```python
from build123d import *

# Parameters (mm, degrees)
SKETCH1_R           = 2.1
SKETCH1_R_2         = 1.5
SKETCH1_W           = 42
SKETCH1_H           = 21
BOSS_EXTRUDE1_DEPTH = 10
BOSS_EXTRUDE2_START = -30
BOSS_EXTRUDE2_DEPTH = 30
SKETCH3_W           = 75
SKETCH3_H           = 8
CUT_EXTRUDE1_DEPTH  = 45
SKETCH4_W           = 7.58
SKETCH4_H           = 21
CUT_EXTRUDE2_DEPTH  = 3


with BuildPart() as part:
    # Sketch1 → Boss-Extrude1 (new body)
    with BuildSketch(Plane(origin=(0, 0, 0), x_dir=(1, 0, 0), z_dir=(0, 1, 0))):
        with BuildLine():
            Line((-100, 32.5), (100, 32.5))
            ThreePointArc((100, 32.5), (132.5, 0), (100, -32.5))
            Line((100, -32.5), (-100, -32.5))
            ThreePointArc((-100, -32.5), (-132.5, 0), (-100, 32.5))
        make_face()
        with Locations(Location((-115.5, 4.9, 0), (0, 0, 270))):
            Circle(SKETCH1_R, mode=Mode.SUBTRACT)
        with Locations(Location((-115.5, -4.9, 0), (0, 0, 270))):
            Circle(SKETCH1_R, mode=Mode.SUBTRACT)
        with Locations(Location((-66.5, -4.9, 0), (0, 0, 270))):
            Circle(SKETCH1_R, mode=Mode.SUBTRACT)
        with Locations(Location((-66.5, 4.9, 0), (0, 0, 270))):
            Circle(SKETCH1_R, mode=Mode.SUBTRACT)
        with Locations(Location((85, 15, 0), (0, 0, 270))):
            Circle(SKETCH1_R_2, mode=Mode.SUBTRACT)
        with Locations(Location((115, 15, 0), (0, 0, 90))):
            Circle(SKETCH1_R_2, mode=Mode.SUBTRACT)
        with Locations(Location((85, -15, 0), (0, 0, 90))):
            Circle(SKETCH1_R_2, mode=Mode.SUBTRACT)
        with Locations(Location((115, -15, 0), (0, 0, 270))):
            Circle(SKETCH1_R_2, mode=Mode.SUBTRACT)
        with Locations((-91, 0)):
            Rectangle(SKETCH1_W, SKETCH1_H, mode=Mode.SUBTRACT)
        Polygon((0, 21.5), (-40, 21.5), (-40, 12), (0, 12), (50, 12), (50, 21.5), align=None, mode=Mode.SUBTRACT)
        Polygon((-50, 4.75), (0, 4.75), (65, 4.75), (65, -4.75), (0, -4.75), (-50, -4.75), align=None, mode=Mode.SUBTRACT)
        Polygon((0, -12), (-40, -12), (-40, -21.5), (0, -21.5), (50, -21.5), (50, -12), align=None, mode=Mode.SUBTRACT)
    extrude(amount=BOSS_EXTRUDE1_DEPTH)

    # Sketch2 → Boss-Extrude2 (add)
    with BuildSketch(Plane(origin=(0, 0, 0), x_dir=(1, 0, 0), z_dir=(0, 1, 0)).offset(BOSS_EXTRUDE2_START)):
        with BuildLine():
            Line((-100, 32.5), (100, 32.5))
            ThreePointArc((100, 32.5), (132.5, 0), (100, -32.5))
            Line((100, -32.5), (-100, -32.5))
            ThreePointArc((-100, -32.5), (-132.5, 0), (-100, 32.5))
        make_face()
        with BuildLine():
            Line((99.668543355, 27.510998447), (-100, 27.510998447))
            ThreePointArc((-100, 27.510998447), (-127.55585262, -0.044854173), (-100, -27.600706793))
            Line((-100, -27.600706793), (100.998461852, -27.600706793))
            ThreePointArc((100.998461852, -27.600706793), (128.562336478, 0.636345006), (99.668543355, 27.510998447))
        make_face(mode=Mode.SUBTRACT)
    extrude(amount=BOSS_EXTRUDE2_DEPTH)

    # Sketch3 → Cut-Extrude1 (cut, symmetric)
    with BuildSketch(Plane.XY):
        with Locations((-57.5, -19)):
            Rectangle(SKETCH3_W, SKETCH3_H)
        with Locations((57.5, -19)):
            Rectangle(SKETCH3_W, SKETCH3_H)
        with Locations((57.5, -4)):
            Rectangle(SKETCH3_W, SKETCH3_H)
        with Locations((-57.5, -4)):
            Rectangle(SKETCH3_W, SKETCH3_H)
    extrude(amount=CUT_EXTRUDE1_DEPTH, both=True, mode=Mode.SUBTRACT)

    # Sketch4 → Cut-Extrude2 (cut)
    with BuildSketch(Plane(origin=(0, 10, 0), x_dir=(1, 0, 0), z_dir=(0, 1, 0))):
        with Locations((-115.79, 0)):
            Rectangle(SKETCH4_W, SKETCH4_H)
        with Locations((-66.21, 0)):
            Rectangle(SKETCH4_W, SKETCH4_H)
    extrude(amount=-CUT_EXTRUDE2_DEPTH, mode=Mode.SUBTRACT)


solid = part.part
```
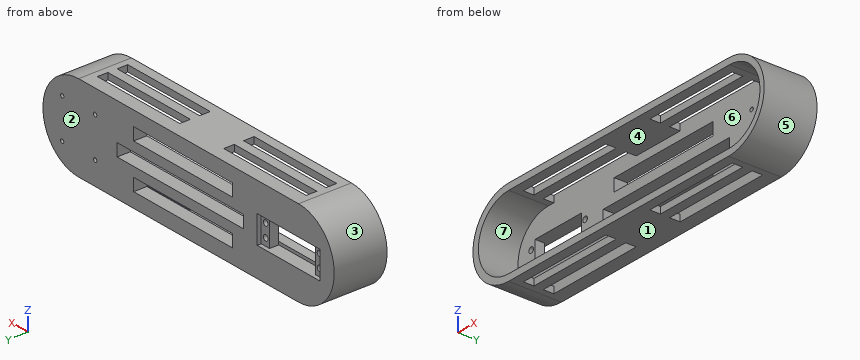
The model under review builds one solid part; all positions refer to its coordinate system, in mm. Face numbers are marked on the shaded views. A direction names the side the tool comes from. Round coordinates to 2 decimals unless told otherwise and drop trailing zeros. Loops run counter-clockwise (first coordinate to the right, second up) from the corner with the lowest first, then second, coordinate; pieces in that order, holes last. Notation, with made-up numbers: (-24, 85) - (32, 85) arc R30 ccw to (32, 109) - close; hole circle Ø6 at (9, 49.25). An arc over 180 degrees is marked (long way). Write each question's results on one line, items separated by ' | '. Start each with the question number.
Q1. Wall thickness on line 1 along Y through (x, z) = (-71, -28); line 2 along Z through (x, y) = (85, 7); line 3 along Z through (x, y) = (-58.5, -14): over which ranges is each line inside the solid? List them lowest first. Write a range as [from, to].
Q2. Draft analysis for pull direction Z (two halves, no side actions). For the marked faces 1, 2, 3 and 4, state which applies: pulls with the +Z half, pulls with the -Z half, needs draft (parallel to the pull), parting line crosses it, or undercut.
Q3. Take a section at C-C on z = 0. Give the boundary of the cut face in (x, y), plus the area to 3 significant figures.
Q4. Take a section at B-B on x = 4.5. Give the boundary of the cut face in (y, z), plus the area to 3 significant figures.
Q5. Insertion check: P1, Ø3, axis at y = 4.5, z = -17.5, coming from the +X side; P2, Ø10, axis at y = -22, z = 23.5, coming from the -X side; P3, Ø2.5, axis at y = -17, z = 29, coming from the +X side. Each pin has a flat end and moves straight along its axis. Give the tip position at first contact, or say it passes through.
Q6. Take a section at A-A on x = 56. Give the boundary of the cut face in (y, z), plus the area to 3 significant figures.
Q7. Tool access review of the marked faces 5, 6 and 7: name each direction out of +Z, -Z, +X, -X, +Y, -Y from which nothing blocks a thin tool from reaching the whole face with its end or side.
Data:
1) line 1: y = [-30, -23], [-15, -8], [0, 10] | line 2: z = [-32.5, -16.5], [-13.5, 13.5], [16.5, 32.5] | line 3: z = [-32.5, -27.51], [27.6, 32.5]
2) face 1: pulls with the -Z half | face 2: needs draft | face 3: parting line crosses it | face 4: undercut
3) outline: (-132.5, -30) - (-127.56, -30) - (-127.56, 0) - (-112, 0) - (-112, 7) - (-119.58, 7) - (-119.58, 10) - (-132.5, 10) - close; (-70, 0) - (-50, 0) - (-50, 10) - (-62.42, 10) - (-62.42, 7) - (-70, 7) - close; (65, 0) - (128.57, 0) - (128.57, -30) - (132.5, -30) - (132.5, 10) - (65, 10) - close | area: 1,300 mm²
4) outline: (-30, -32.5) - (10, -32.5) - (10, -21.5) - (0, -21.5) - (0, -27.51) - (-30, -27.51) - close; (-30, 27.6) - (0, 27.6) - (0, 21.5) - (10, 21.5) - (10, 32.5) - (-30, 32.5) - close; (0, -12) - (10, -12) - (10, -4.75) - (0, -4.75) - close; (0, 4.75) - (10, 4.75) - (10, 12) - (0, 12) - close | area: 662 mm²
5) P1: stops at x = 128.29 | P2: stops at x = -126.72 | P3: stops at x = 116.92
6) outline: (-30, -32.5) - (-23, -32.5) - (-23, -27.51) - (-30, -27.51) - close; (-30, 27.6) - (-23, 27.6) - (-23, 32.5) - (-30, 32.5) - close; (-15, -32.5) - (-8, -32.5) - (-8, -27.51) - (-15, -27.51) - close; (-15, 27.6) - (-8, 27.6) - (-8, 32.5) - (-15, 32.5) - close; (0, -32.5) - (10, -32.5) - (10, -4.75) - (0, -4.75) - close; (0, 4.75) - (10, 4.75) - (10, 32.5) - (0, 32.5) - close | area: 693 mm²
7) face 5: +X, +Y, -Y | face 6: none | face 7: -Y
